The figure shows three views and two pictorial views of one solid part (mm, origin at its lowest corner). Answer the questions. Coordinates: 2 decimals unless noted, no trailing zeros. Order: outer loops, then holes, each group sorted by start corner. A loop starts at its lowest first (then second) coordinate and runs counter-clockwise, first axis right, second up.
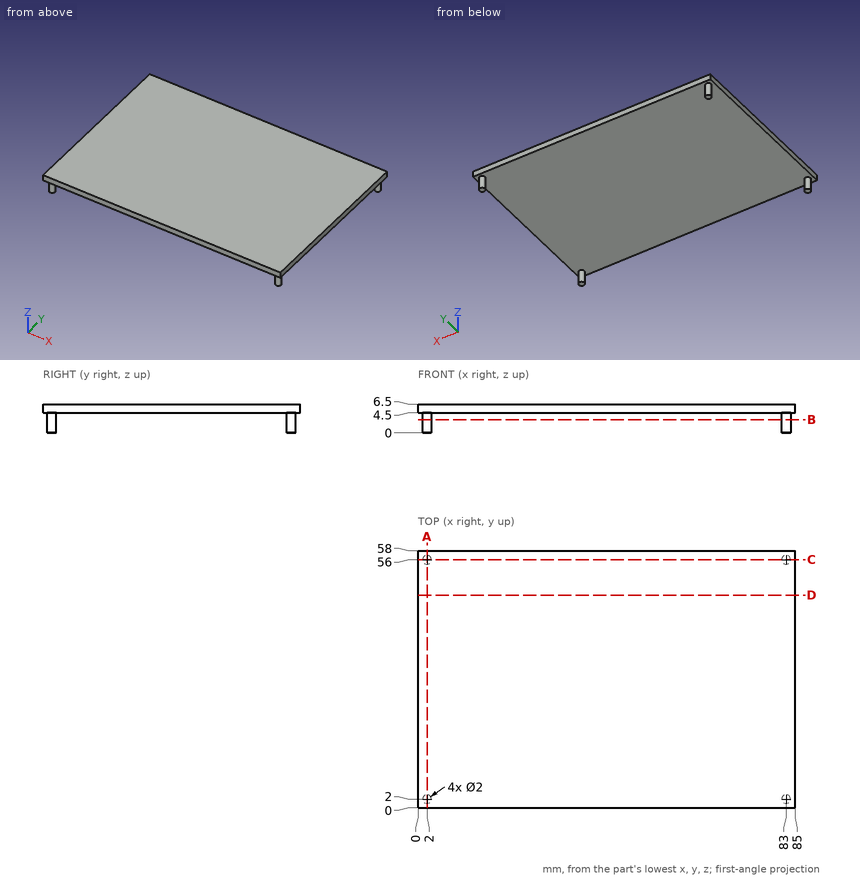
1) A cutting plane is placed at C-C, the plane y = 56. Write down the section's boundary in (x, z).
2) This flat-tipped pin is pushed along its axis until it touches: P1, Ø3, axis at x = 55.5, y = 23, coming from the -Z side. Where does it stop, or does it pass through?
3) A straight line is drawn through the part: probe 1 along Z at (x, y) = (5, 9). Find the intervals that lie inside material, in ascending order.
4) A cutting plane is placed at D-D, the plane y = 48. Write down the section's boundary in (x, z), plus the area to 3 significant figures.
5) A cutting plane is placed at B-B, the plane z = 3. Write down the section's boundary in (x, y).
6) A cutting plane is placed at A-A, the plane x = 2. Write down the section's boundary in (y, z).
Working result:
1. outline: (0, 4.5) - (1, 4.5) - (1, 0) - (3, 0) - (3, 4.5) - (82, 4.5) - (82, 0) - (84, 0) - (84, 4.5) - (85, 4.5) - (85, 6.5) - (0, 6.5) - close
2. P1: stops at z = 4.5
3. probe 1: z = 4.5 to 6.5
4. outline: (0, 4.5) - (85, 4.5) - (85, 6.5) - (0, 6.5) - close
4. area: 170 mm2
5. outline: circle Ø2 at (2, 2); circle Ø2 at (2, 56); circle Ø2 at (83, 2); circle Ø2 at (83, 56)
6. outline: (0, 4.5) - (1, 4.5) - (1, 0) - (3, 0) - (3, 4.5) - (55, 4.5) - (55, 0) - (57, 0) - (57, 4.5) - (58, 4.5) - (58, 6.5) - (0, 6.5) - close
